The model under review builds one solid part; all positions refer to its coordinate system, in mm. A direction names the side the tool comes from. Coordinates: 2 decimals unless noted, no trailing zeros. Order: outer loops, then holes, each group sorted by start corner. A loop starts at its lowest first (then second) coordinate and runs counter-clockwise, first axis right, second up. Notation, with made-up numbers: (14.25, 70) -> (50.25, 70) arc R15 ccw to (50.25, 87) -> close; hole circle Ø9 at (61.25, -15). An arc over 180 degrees is marked (long way). Use CSV: the item, a comma, the result in double quotes. Start each with the question number.
```python
from build123d import *

# Parameters (mm, degrees)
BOSS_EXTRU_2_DEPTH      = 5
ESQUISSE1_4_W           = 71
ESQUISSE1_4_H           = 24
ENL_V_MAT_EXTRU_2_DEPTH = 7
ESQUISSE1_5_R           = 3
ESQUISSE1_5_R_2         = 1.25
ENL_V_MAT_EXTRU_3_DEPTH = 10


with BuildPart() as part:
    # Esquisse1 → Boss.-Extru.2 (new body)
    with BuildSketch(Plane.XY):
        Polygon((-79.904859092, -61.651270208), (-79.904859092, -46.651270208), (80.095140908, -46.651270208), (80.095140908, -61.651270208), (75.095140908, -61.651270208), (75.095140908, -78.221270208), (80.095140908, -78.221270208), (80.095140908, -93.221270208), (-79.904859092, -93.221270208), (-79.904859092, -78.221270208), (-74.904859092, -78.221270208), (-74.904859092, -61.651270208), align=None)
    extrude(amount=BOSS_EXTRU_2_DEPTH)

    # Esquisse1_4 → Enl_v. mat.-Extru.2 (cut)
    with BuildSketch(Plane.XY):
        with Locations((-19.404859092, -66.651270208)):
            Rectangle(ESQUISSE1_4_W, ESQUISSE1_4_H)
    extrude(amount=ENL_V_MAT_EXTRU_2_DEPTH, mode=Mode.SUBTRACT)

    # Esquisse1_5 → Enl_v. mat.-Extru.3 (cut)
    with BuildSketch(Plane.XY):
        with Locations(Location((40.095140908, -61.651270208, 0), (0, 0, 180))):
            Circle(ESQUISSE1_5_R)
        with Locations(Location((40.095140908, -76.651270208, 0), (0, 0, 180))):
            Circle(ESQUISSE1_5_R)
        with Locations(Location((55.095140908, -61.651270208, 0), (0, 0, 180))):
            Circle(ESQUISSE1_5_R)
        with Locations(Location((55.095140908, -76.651270208, 0), (0, 0, 180))):
            Circle(ESQUISSE1_5_R)
        with Locations(Location((13.095140908, -50.651270208, 0), (0, 0, 180))):
            Circle(ESQUISSE1_5_R_2)
        with Locations(Location((-26.904859092, -50.651270208, 0), (0, 0, 180))):
            Circle(ESQUISSE1_5_R_2)
        with Locations(Location((-6.904859092, -90.651270208, 0), (0, 0, 180))):
            Circle(ESQUISSE1_5_R_2)
    extrude(amount=ENL_V_MAT_EXTRU_3_DEPTH, mode=Mode.SUBTRACT)


solid = part.part
```
Q1. Add section B-B, the plane x = -23.5. State the section outline as (y, z) points.
Q2. Add section A-A, the plane y = -69.5. State the section outline as (x, z) points, then the cut area to 3 significant figures.
Q3. Add section C-C, the plane z = 3.3. State how many separate pieces and enclosed holes the cut face has, then the cut area to 3 significant figures.
Q4. For faces 5 (the flat face through (-77, -61.651, 2)), 6 (the flat face through (78, -78.221, 2)), 7 (the flat face through (-20, -78.651, 2)), 8 (the flat face through (80.095, -54, 2)), 9 (the flat face through (1, -80, 0)), list the 3-axis set-ups (+Z, -Z, +X, -X, +Y, -Y) from which the entire face can be reached by the end or side of a thin tool; tool diameter is ignored.
Q5. Draft analysis for pull direction X (two halves, no side actions). For faces 1 (the flat face through (-54.905, -67, 2)), 2 (the cylindrical face through (53.48, -64.18, 2.46)), 3 (the flat face through (75.095, -70, 2)), 4 (the flat face through (-79.905, -86, 2)), state which applies: +X half, -X half, draft (parallel to the pull), parting line (faces both ways), or undercut.
Q6. Clearance check with flat-ended pins moving along their axes: pin 1 Ø5 at (x, y) = (55.1, -61.65) entering from +Z; pin 2 Ø1.5 at (y, z) = (-68.5, 3.5) entering from +X. State where each tip first meets the part, or that it passes through.
Q7. To check wall thickness, follow probe 1 along X at (y, z) = (-61.5, 0.8); probe 2 along Y at (x, z) = (-5, 0.85); probe 3 along Y at (x, z) = (-7.5, 2.8). State the ranges of each line that lie inside material, in increasing order.
Answer block:
1,outline,"(-93.22, 0) -> (-78.65, 0) -> (-78.65, 5) -> (-93.22, 5) -> close; (-54.65, 0) -> (-46.65, 0) -> (-46.65, 5) -> (-54.65, 5) -> close"
2,outline,"(-74.9, 0) -> (-54.9, 0) -> (-54.9, 5) -> (-74.9, 5) -> close; (16.1, 0) -> (75.1, 0) -> (75.1, 5) -> (16.1, 5) -> close"
2,area,"395 mm²"
3,separate pieces,"1"
3,enclosed holes,"8"
3,area,"5,450 mm²"
4,face 5,"+Z, -Z, -X"
4,face 6,"+Z, -Z, +X"
4,face 7,"+Z, -Z"
4,face 8,"+Z, -Z, +X, +Y, -Y"
4,face 9,"-Z, +X, -X, +Y, -Y"
5,face 1,"undercut"
5,face 2,"undercut"
5,face 3,"+X half"
5,face 4,"-X half"
6,pin 1,"passes through"
6,pin 2,"stops at x = 75.1"
7,probe 1,"x = -79.9 to -54.9, 16.1 to 37.1, 43.09 to 52.1, 58.09 to 80.1"
7,probe 2,"y = -93.22 to -78.65, -54.65 to -46.65"
7,probe 3,"y = -93.22 to -91.75, -89.55 to -78.65, -54.65 to -46.65"
